CAD build for the part. Positions are in the model's coordinates, mm. Round coordinates to 2 decimals unless told otherwise and drop trailing zeros. Loops run counter-clockwise (first coordinate to the right, second up) from the corner with the lowest first, then second, coordinate; pieces in that order, holes last.
from build123d import *

# Parameters (mm, degrees)
SKETCH1_W           = 73.025
SKETCH1_H           = 215.9
BOSS_EXTRUDE1_DEPTH = 3.175
SKETCH2_R           = 2.667
CUT_EXTRUDE1_DEPTH  = 3.175


with BuildPart() as part:
    # Sketch1 → Boss-Extrude1 (new body)
    with BuildSketch(Plane.XY):
        Rectangle(SKETCH1_W, SKETCH1_H)
    extrude(amount=BOSS_EXTRUDE1_DEPTH)

    # Sketch2 → Cut-Extrude1 (cut)
    with BuildSketch(Plane.XY.offset(3.175)):
        with Locations((-23.8125, -69.85)):
            Circle(SKETCH2_R)
        with Locations((-23.8125, -82.55)):
            Circle(SKETCH2_R)
        with Locations((-23.8125, -95.25)):
            Circle(SKETCH2_R)
        with Locations(Location((-23.8125, 95.25, 0), (0, 0, 180))):
            Circle(SKETCH2_R)
        with Locations(Location((-23.8125, 82.55, 0), (0, 0, 180))):
            Circle(SKETCH2_R)
        with Locations(Location((-23.8125, 69.85, 0), (0, 0, 180))):
            Circle(SKETCH2_R)
        with Locations((23.8125, 95.25)):
            Circle(SKETCH2_R)
        with Locations((23.8125, 82.55)):
            Circle(SKETCH2_R)
        with Locations((23.8125, 69.85)):
            Circle(SKETCH2_R)
        with Locations(Location((23.8125, -95.25, 0), (0, 0, 180))):
            Circle(SKETCH2_R)
        with Locations(Location((23.8125, -82.55, 0), (0, 0, 180))):
            Circle(SKETCH2_R)
        with Locations(Location((23.8125, -69.85, 0), (0, 0, 180))):
            Circle(SKETCH2_R)
    extrude(amount=-CUT_EXTRUDE1_DEPTH, mode=Mode.SUBTRACT)


solid = part.part
Item 1: Cut at B-B (y = -95.25). List the corners of the cut face in (x, z) (1 decimal).
Verdict:
outline: (-36.5, 0) - (-26.5, 0) - (-26.5, 3.2) - (-36.5, 3.2) - close; (-21.1, 0) - (21.1, 0) - (21.1, 3.2) - (-21.1, 3.2) - close; (26.5, 0) - (36.5, 0) - (36.5, 3.2) - (26.5, 3.2) - close
Item 2: Cut at A-A (z = 0.85). State how many separate pieces and enclosed holes the cut face has, plus the area to 3 significant figures.
Verdict:
separate pieces: 1
enclosed holes: 12
area: 15,500 mm2
Item 3: Mould opens along Y. For faces 1 (the cylindrical face through (-21.696, 84.173, 1.61)), 2 (the flat face through (-1, 2, 3.175)) say: released by +Y, released by -Y, zero draft, split by the parting line, or undercut.
Verdict:
face 1: undercut
face 2: zero draft
